Design review of the part shown in the three views and the two pictorial views. Dimensions are in mm from the part's minimum x, y and z. Give positions to 0.01 mm unless a question says otherwise; leave off trailing zeros. Loops run counter-clockwise (first coordinate to the right, second up) from the corner with the lowest first, then second, coordinate; pieces in that order, holes last. Notation, with made-up numbers: (21.5, -21.75) - (32.5, -21.75) arc R22 cw to (32.5, 13.25) - close; hole circle Ø1 at (-26.5, 89.5). An arc over 180 degrees is marked (long way). Answer in a Markdown table with one row per item.
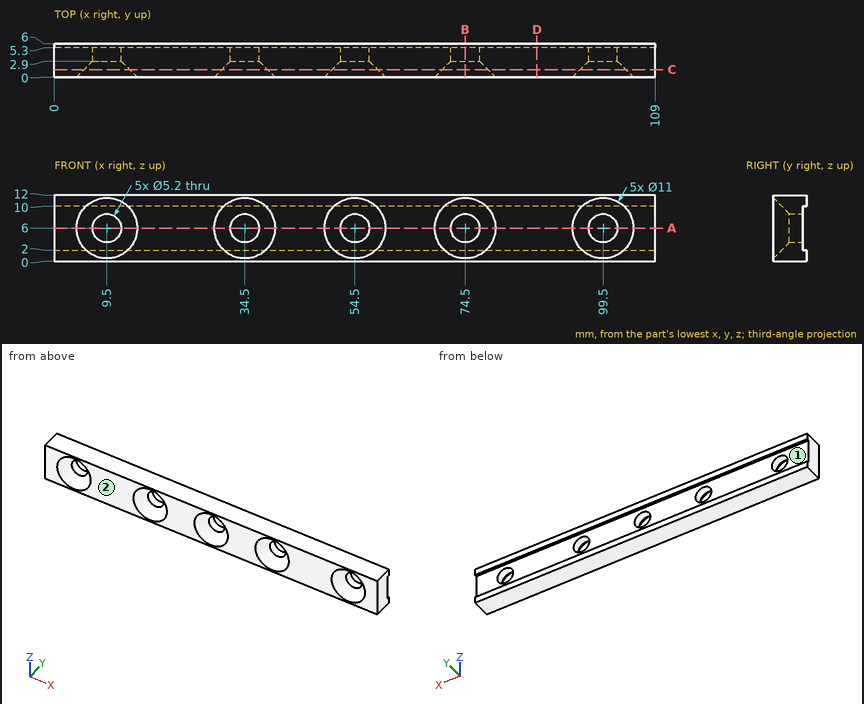
1. We need section A-A, the plane z = 6. Count the separate pieces of the cut face and the enclosed holes in it, and give its area (3 significant figures).
Values:
| item | result |
|---|---|
| separate pieces | 6 |
| enclosed holes | 0 |
| area | 398 mm^2 |
2. We need section B-B, the plane x = 74.5. Give the boundary of the cut face in (y, z).
Values:
| item | result |
|---|---|
| outline | (0, 0) - (6, 0) - (6, 2) - (5.3, 2) - (5.3, 3.4) - (2.9, 3.4) - (0, 0.5) - close; (0, 11.5) - (2.9, 8.6) - (5.3, 8.6) - (5.3, 10) - (6, 10) - (6, 12) - (0, 12) - close |
3. Wall thickness on line 1 (X direction, y = 3.6, z = 6); line 2 (Z direction, x = 54.5, y = 4.4); line 3 (X direction, y = 2.2, z = 5.25): over which ranges is each line inside the solid? List them lowest first. Write a range as [from, to].
Values:
| item | result |
|---|---|
| line 1 | x = [0, 6.9], [12.1, 31.9], [37.1, 51.9], [57.1, 71.9], [77.1, 96.9], [102.1, 109] |
| line 2 | z = [0, 3.4], [8.6, 12] |
| line 3 | x = [0, 6.29], [12.71, 31.29], [37.71, 51.29], [57.71, 71.29], [77.71, 96.29], [102.71, 109] |
4. Mouldability with a two-part tool opening along Z and no side actions: class the marked faces 1 and 2 as released by +Z, released by -Z, zero draft, split by the parting line, or undercut.
Values:
| item | result |
|---|---|
| face 1 | undercut |
| face 2 | zero draft |
5. We need section C-C, the plane y = 1.35. Give the boundary of the cut face in (x, z).
Values:
| item | result |
|---|---|
| outline | (0, 0) - (109, 0) - (109, 12) - (0, 12) - close; hole circle Ø8.3 at (9.5, 6); hole circle Ø8.3 at (34.5, 6); hole circle Ø8.3 at (54.5, 6); hole circle Ø8.3 at (74.5, 6); hole circle Ø8.3 at (99.5, 6) |
6. Clearance check with flat-ended pins moving along their axes: pin 1 (6.5 mm diameter, centred on x = 39.5, z = 6, fed in from +Y); pin 2 (7 mm diameter, centred on x = 34.5, z = 6, fed in from -Y); pin 3 (6 mm diameter, centred on x = 99.5, z = 6, fed in from -Y). State where each tip first meets the part, or that it passes through.
Values:
| item | result |
|---|---|
| pin 1 | stops at y = 5.3 |
| pin 2 | stops at y = 2 |
| pin 3 | stops at y = 2.5 |
7. We need section D-D, the plane x = 87.5. Give the boundary of the cut face in (y, z).
Values:
| item | result |
|---|---|
| outline | (0, 0) - (6, 0) - (6, 2) - (5.3, 2) - (5.3, 10) - (6, 10) - (6, 12) - (0, 12) - close |
